Part model, mm, in its own coordinate system. A direction names the side the tool comes from. Give positions to 0.01 mm unless a question says otherwise; leave off trailing zeros. Write each loop counter-clockwise with the first axis right and the second up, starting at its lowest first coordinate (ties: lowest second). Pieces come first, ordered by that corner, then holes. Notation, with made-up numbers: (-16, 33.25) - (2, 33.25) arc R25 ccw to (2, 49.25) - close; hole circle Ø8 at (70.25, 18.25). An arc over 180 degrees is marked (long way). Answer in a Markdown table with one row per item. Add a question column.
1. Pull direction Y, two halves, no side cores. Call faces 4 (the flat face through (-31, 45, 0)), 5 (the flat face through (-32.5, 20, 0)), 6 (the flat face through (18, 28.55, 0)), 7 (the flat face through (-29.5, -27, 0)): released by +Y, released by -Y, zero draft, split by the parting line, or undercut.
2. Which spindle directions (+Z, -Z, +X, -X, +Y, -Y) get a long thin tool onto all of the face, cutting with end or side? Do faces 1 (the flat face through (-2.5, -58, 0)), 2 (the flat face through (-31, -35, 0)), 3 (the flat face through (29.5, 27, 0)). Say none if no direction does.
3. Probe line 1 along Y through (x, z) = (-25, 1.1); line 2 along X through (y, z) = (57.5, -1.5); line 3 along X through (y, z) = (46.5, -1.6). List the from-to ranges inside material, lowest first.
4. Band-saw the part on C-C on z = 0.05. State how many separate pieces and enclosed holes the cut face has, plus the area to 3 significant figures.
5. Band-saw the part on A-A on y = 11.45. Write the cut outline in (x, z).
6. Band-saw the part on D-D on y = -8. Write the cut outline in (x, z).
7. Band-saw the part on B-B on y = 53.55. Write the cut outline in (x, z), plus the area to 3 significant figures.
8. Drop flat-ended pins along their axis: pin 1 Ø2 at (y, z) = (-33, -0.5) entering from -X; pin 2 Ø2 at (y, z) = (-25.5, 1.5) entering from +X; pin 3 Ø1.5 at (y, z) = (26, -1) entering from +X; pin 4 Ø0.9 at (x, z) = (-30.5, -1) entering from +Y. Give the stop position or say it passes through.
Autodesk Inventor part; units mm, degrees
sketch "Эскиз1" plane through (0, 0, 0) normal (0, 0, 1) x (1, 0, 0)
  line L0 (-29.5, -65) -> (29.5, -65)
  line L1 (29.5, -65) -> (29.5, 65)
  line L2 (29.5, 65) -> (-29.5, 65)
  line L3 (-29.5, 65) -> (-29.5, -65)
  line L4 (-29.5, -65) -> (29.5, 65) construction
  line L5 (29.5, -65) -> (-29.5, 65) construction
  point P0 (0, 0)
  dimension "d0" = 59
  dimension "d1" = 130
extrude "Выдавливание1" add sketch "Эскиз1" along normal mid plane 4
sketch "Эскиз3" plane through (-29.5, -65, 2) normal (-1, 0, 0) x (0, 0, 1)
  line L0 (-4, 0) -> (-4, 130)
  line L1 (0, 0) -> (0, 130)
  line L2 (-4, 100) -> (0, 100)
  line L3 (0, 100) -> (0, 110)
  line L4 (0, 110) -> (-4, 110)
  line L5 (-4, 110) -> (-4, 100)
  line L6 (-4, 130) -> (0, 130)
  line L7 (-4, 90) -> (0, 90)
  line L8 (0, 90) -> (0, 80)
  line L9 (0, 80) -> (-4, 80)
  line L10 (-4, 80) -> (-4, 90)
  line L11 (-4, 65) -> (0, 65) construction
  line L12 (-4, 30) -> (0, 30)
  line L13 (0, 30) -> (0, 20)
  line L14 (0, 20) -> (-4, 20)
  line L15 (-4, 20) -> (-4, 30)
  line L16 (-4, 40) -> (0, 40)
  line L17 (0, 40) -> (0, 50)
  line L18 (0, 50) -> (-4, 50)
  line L19 (-4, 50) -> (-4, 40)
  point P0 (-2, 65)
  point P1 (0, 30)
  point P2 (0, 40)
  point P3 (0, 90)
  point P4 (0, 100)
  dimension "d18" = 10
  dimension "d19" = 10
  dimension "d20" = 20
  dimension "d21" = 10
extrude "Выдавливание3" add sketch "Эскиз3" along normal blind 3 contours L0 L12 L1 L14 | L0 L18 L1 L16 | L0 L7 L1 L9 | L0 L4 L1 L2
mirror "Зеркальное отражение2" about plane through (0, 0, 0) normal (1, 0, 0) of "Выдавливание3"
sketch "Эскиз4" plane through (0, 0, 2) normal (0, 0, 1) x (1, 0, 0)
  line L0 (-15.4, 31.45) -> (-15.4, 28.55)
  line L1 (-29.5, 28.55) -> (-29.5, 31.45)
  line L2 (-22.5, 32.8) -> (-20.7, 32.8)
  line L3 (-22.5, 27.2) -> (-20.7, 27.2)
  line L4 (-29.5, 30) -> (-15.4, 30)
  line L5 (-20.7, 27.2) -> (-20.7, 28.55)
  line L6 (-22.5, 31.45) -> (-22.5, 32.8)
  line L7 (-20.7, 32.8) -> (-20.7, 31.45)
  line L8 (-22.5, 28.55) -> (-22.5, 27.2)
  line L9 (-29.5, 31.45) -> (-22.5, 31.45)
  line L10 (-20.7, 31.45) -> (-15.4, 31.45)
  line L11 (-15.4, 28.55) -> (-20.7, 28.55)
  line L12 (-22.5, 28.55) -> (-29.5, 28.55)
  line L13 (-29.5, 35) -> (-29.5, 25)
  line L14 (0, 3.054) -> (0, -3.054) construction
  line L15 (-15.3649, 0) -> (15.3649, 0)
  line L16 (-15.4, -31.45) -> (-15.4, -28.55)
  line L17 (-29.5, -28.55) -> (-29.5, -31.45)
  line L18 (-22.5, -32.8) -> (-20.7, -32.8)
  line L19 (-22.5, -27.2) -> (-20.7, -27.2)
  line L20 (-29.5, -30) -> (-15.4, -30)
  line L21 (-20.7, -27.2) -> (-20.7, -28.55)
  line L22 (-22.5, -31.45) -> (-22.5, -32.8)
  line L23 (-20.7, -32.8) -> (-20.7, -31.45)
  line L24 (-22.5, -28.55) -> (-22.5, -27.2)
  line L25 (-29.5, -31.45) -> (-22.5, -31.45)
  line L26 (-20.7, -31.45) -> (-15.4, -31.45)
  line L27 (-15.4, -28.55) -> (-20.7, -28.55)
  line L28 (-22.5, -28.55) -> (-29.5, -28.55)
  line L29 (-29.5, -35) -> (-29.5, -25)
  line L30 (0, -3.054) -> (0, 3.054) construction
  line L31 (15.4, 31.45) -> (15.4, 28.55)
  line L32 (29.5, 28.55) -> (29.5, 31.45)
  line L33 (22.5, 32.8) -> (20.7, 32.8)
  line L34 (22.5, 27.2) -> (20.7, 27.2)
  line L35 (29.5, 30) -> (15.4, 30)
  line L36 (20.7, 27.2) -> (20.7, 28.55)
  line L37 (22.5, 31.45) -> (22.5, 32.8)
  line L38 (20.7, 32.8) -> (20.7, 31.45)
  line L39 (22.5, 28.55) -> (22.5, 27.2)
  line L40 (29.5, 31.45) -> (22.5, 31.45)
  line L41 (20.7, 31.45) -> (15.4, 31.45)
  line L42 (15.4, 28.55) -> (20.7, 28.55)
  line L43 (22.5, 28.55) -> (29.5, 28.55)
  line L44 (29.5, 35) -> (29.5, 25)
  line L45 (20.7, -27.2) -> (20.7, -28.55)
  line L46 (22.5, -27.2) -> (20.7, -27.2)
  line L47 (22.5, -28.55) -> (22.5, -27.2)
  line L48 (20.7, -31.45) -> (15.4, -31.45)
  line L49 (20.7, -32.8) -> (20.7, -31.45)
  line L50 (22.5, -32.8) -> (20.7, -32.8)
  line L51 (22.5, -31.45) -> (22.5, -32.8)
  line L52 (29.5, -30) -> (15.4, -30)
  line L53 (22.5, -28.55) -> (29.5, -28.55)
  line L54 (29.5, -28.55) -> (29.5, -31.45)
  line L55 (29.5, -31.45) -> (22.5, -31.45)
  line L56 (15.4, -31.45) -> (15.4, -28.55)
  line L57 (15.4, -28.55) -> (20.7, -28.55)
  point P0 (0, 0)
  point P1 (0, 0)
  point P2 (29.5, -25)
  dimension "d26" = 2.9
  dimension "d31" = 1.8
  dimension "d32" = 1.35
  dimension "d33" = 7
  dimension "d34" = 5.3
  dimension "d35" = 2.9
extrude "Выдавливание4" cut sketch "Эскиз4" against normal up to surface (4 mm away)
sketch "Эскиз5" plane through (0, 0, 2) normal (0, 0, 1) x (1, 0, 0)
  line L0 (29.5, 65) -> (-29.5, 65) construction
  line L1 (2.5, 65) -> (-2.5, 65)
  line L2 (-2.5, 65) -> (-2.5, 50)
  line L3 (-2.5, 50) -> (2.5, 50)
  line L4 (2.5, 50) -> (2.5, 65)
  line L5 (-2.9793, 0) -> (2.9793, 0) construction
  line L6 (29.5, -65) -> (-29.5, -65) construction
  line L7 (-2.5, -65) -> (-2.5, -50)
  line L8 (-2.5, -50) -> (2.5, -50)
  line L9 (2.5, -50) -> (2.5, -65)
  line L10 (-2.5, -65) -> (2.5, -65)
  line L11 (-29.5, -65) -> (29.5, -65)
  point P0 (0, 0)
  point P1 (0, 65)
  point P2 (0, 0)
  dimension "d38" = 5
  dimension "d39" = 15
extrude "Выдавливание5" cut sketch "Эскиз5" against normal up to surface (4 mm away)
fillet "Сопряжение1" radius 2 8 edges at (2.5, 50, 0) (-2.5, 50, 0) (-2.5, -50, 0) (2.5, -50, 0) (2.5, 65, 0) (-2.5, 65, 0) (2.5, -65, 0) (-2.5, -65, 0)
sketch "Эскиз8" plane through (0, 0, 2) normal (0, 0, 1) x (1, 0, 0)
  circle A0 centre (-21.05, 11.45) radius 1.5
  circle A1 centre (21.05, 11.45) radius 1.5
  circle A2 centre (-21.05, 53.55) radius 1.5
  circle A3 centre (21.05, 53.55) radius 1.5
  circle A4 centre (21.05, -11.45) radius 1.5
  circle A5 centre (-21.05, -11.45) radius 1.5
  circle A6 centre (-21.05, -53.55) radius 1.5
  circle A7 centre (21.05, -53.55) radius 1.5
  point P0 (0, 0)
extrude "Выдавливание8" cut sketch "Эскиз8" against normal up to surface (4 mm away)
properties part number "Фанерка ерпления колонок"
Values:
| question | item | result |
|---|---|---|
| 1 | face 4 | released by +Y |
| 1 | face 5 | zero draft |
| 1 | face 6 | undercut |
| 1 | face 7 | undercut |
| 2 | face 1 | +Z, -Z, -Y |
| 2 | face 2 | +Z, -Z, -X |
| 2 | face 3 | +Z, -Z, +X |
| 3 | line 1 | y = -65 to -31.45, -28.55 to 28.55, 31.45 to 65 |
| 3 | line 2 | x = -29.5 to -2.5, 2.5 to 29.5 |
| 3 | line 3 | x = -29.5 to 29.5 |
| 4 | separate pieces | 1 |
| 4 | enclosed holes | 8 |
| 4 | area | 7,520 mm² |
| 5 | outline | (-29.5, -2) - (-22.55, -2) - (-22.55, 2) - (-29.5, 2) - close; (-19.55, -2) - (19.55, -2) - (19.55, 2) - (-19.55, 2) - close; (22.55, -2) - (29.5, -2) - (29.5, 2) - (22.55, 2) - close |
| 6 | outline | (-29.5, -2) - (29.5, -2) - (29.5, 2) - (-29.5, 2) - close |
| 7 | outline | (-29.5, -2) - (-22.55, -2) - (-22.55, 2) - (-29.5, 2) - close; (-19.55, -2) - (-2.5, -2) - (-2.5, 2) - (-19.55, 2) - close; (2.5, -2) - (19.55, -2) - (19.55, 2) - (2.5, 2) - close; (22.55, -2) - (29.5, -2) - (29.5, 2) - (22.55, 2) - close |
| 7 | area | 192 mm² |
| 8 | pin 1 | stops at x = -29.5 |
| 8 | pin 2 | stops at x = 32.5 |
| 8 | pin 3 | stops at x = 29.5 |
| 8 | pin 4 | stops at y = 45 |
